Autodesk Inventor part; units mm, degrees
ref_plane "YZ Plane" through (0, 0, 0) normal (1, 0, 0) x (0, 1, 0)
ref_plane "XZ Plane" through (0, 0, 0) normal (0, 1, 0) x (-1, 0, 0)
ref_plane "XY Plane" through (0, 0, 0) normal (0, 0, 1) x (1, 0, 0)
sketch "Sketch1" plane through (0, 0, 0) normal (0, 0, 1) x (1, 0, 0)
  circle A0 centre (0, 0) radius 2.3241
  line L0 (0, 0) -> (12.7, 0)
  circle A1 centre (12.7, 0) radius 2.3241
  line L1 (0, 0) -> (12.7, 0) construction
  line L2 (0, -6.35) -> (12.7, -6.35)
  line L3 (12.7, 6.35) -> (0, 6.35)
  arc A2 (0, 6.35) -> (0, -6.35) centre (0, 0) ccw
  arc A3 (12.7, -6.35) -> (12.7, 6.35) centre (12.7, 0) ccw
  point P0 (6.35, 0)
  dimension "d0" = 4.6482
  dimension "d1" = 12.7
  dimension "d2" = 4.6482
  dimension "d3" = 12.7
extrude "Extrusion1" add sketch "Sketch1" along normal blind 12.7
sketch "Sketch2" plane through (0, 0, 0) normal (0, 0, -1) x (-1, 0, 0)
  circle A0 centre (-12.7, 0) radius 2.3241
  circle A1 centre (0, 0) radius 2.3241
  circle A2 centre (-12.7, 0) radius 4.1275
  circle A3 centre (0, 0) radius 4.1275
  dimension "d6" = 8.255
  dimension "d7" = 8.255
extrude "Extrusion2" cut sketch "Sketch2" against normal blind 2.54
sketch "Sketch3" plane through (0, 0, 12.7) normal (0, 0, 1) x (1, 0, 0)
  arc A0 (0, 6.35) -> (0, -6.35) centre (0, 0) ccw
  arc A1 (12.7, -6.35) -> (12.7, 6.35) centre (12.7, 0) ccw
  line L0 (12.7, 6.35) -> (0, 6.35)
  arc A2 (0, 6.35) -> (0, -6.35) centre (0, 0) ccw
  line L1 (0, -6.35) -> (12.7, -6.35)
  circle A3 centre (0, 0) radius 2.3241
  circle A4 centre (12.7, 0) radius 2.3241
  line L2 (19.05, 0) -> (19.05, 38.1)
  line L3 (-6.35, 0) -> (-6.35, 38.1)
  arc A5 (0, 6.35) -> (0, -6.35) centre (0, 0) ccw
  line L4 (-6.35, 38.1) -> (19.05, 38.1)
  line L5 (-6.35, 38.1) -> (-69.85, 38.1)
  line L6 (-6.35, 38.1) -> (-72.261, 62.0897)
  line L7 (-72.261, 62.0897) -> (-72.261, 49.3897)
  arc A6 (-6.35, 0) -> (-72.261, 49.3897) centre (-100.4419, -56.8924) ccw
  line L8 (-34.5064, 31.0993) -> (-34.5064, 48.3481)
  line L9 (-45.0661, 38.1) -> (-45.0661, 52.1915)
  point P0 (0, 6.35)
  point P1 (-34.5064, 38.1)
  dimension "d10" = 38.1
  dimension "d14" = 63.5
  dimension "d15" = 20
  dimension "d16" = 12.7
extrude "Extrusion3" add sketch "Sketch3" against normal up to surface (12.7 mm away) contours A0 L3 L4 L2 A1 L0 | A6 L8 L5 L3 | L5 L8 L6
fillet "Fillet1" radius 6.35 1 edges at (19.05, 38.1, 6.35)
fillet "Fillet2" radius 101.6 1 edges at (-6.35, 38.1, 6.35)
extrude "Extrusion7" add sketch "Sketch3" against normal blind 12.7 contours A0 L3 L4 L2 A1 L0 | A6 L8 L5 L3 | A6 L5 L8 | L5 L9 L6 L8
fillet "Fillet3" radius 6.35 3 edges at (-45.0661, 52.1915, 6.35) (-45.0661, 38.1, 6.35) (19.05, 38.1, 6.35)
sketch "Sketch6" plane through (0, 0, 12.7) normal (0, 0, 1) x (1, 0, 0)
  line L0 (-36.5443, 49.0898) -> (-23.1844, 44.2272)
  line L1 (-26.9453, 41.2324) -> (-18.0387, 37.9907)
  arc A0 (-23.1844, 44.2272) -> (11.5648, 38.1) centre (11.5648, 139.7) ccw
  arc A1 (-18.0387, 37.9907) -> (5.1275, 33.9059) centre (5.1275, 101.6392) ccw
  arc A2 (-36.5443, 49.0898) -> (-45.0661, 43.1228) centre (-38.7161, 43.1228) ccw
  arc A3 (-26.9453, 41.2324) -> (-32.6265, 37.2544) centre (-28.3931, 37.2544) ccw
  arc A4 (-45.0661, 41.681) -> (-42.0862, 36.2991) centre (-38.7161, 41.681) ccw
  arc A5 (-32.6265, 36.2932) -> (-30.6399, 32.7052) centre (-28.3932, 36.2932) ccw
  line L2 (-45.0661, 41.681) -> (-45.0661, 43.1228)
  line L3 (-32.6265, 36.2932) -> (-32.6265, 37.2544)
  arc A6 (-6.35, 0) -> (0, -6.35) centre (0, 0) ccw
  arc A7 (-6.8158, 8.5058) -> (-30.6399, 32.7052) centre (-69.5437, -29.4224) ccw
  arc A8 (12.7, -6.35) -> (19.05, 0) centre (12.7, 0) ccw
  line L4 (-6.8158, 8.5058) -> (10.1176, 8.5058)
  line L5 (10.1176, 8.5058) -> (10.1176, 30.026)
  line L6 (12.7, 38.1) -> (11.5648, 38.1)
  line L7 (5.1275, 33.9059) -> (5.8843, 33.9059)
  arc A9 (10.1176, 30.026) -> (5.8843, 33.9059) centre (5.8784, 29.65) ccw
  circle A10 centre (-38.7161, 43.1228) radius 3.5825
  line L8 (-30.6399, 32.7052) -> (-41.3753, 40.7221)
  line L9 (-37.1542, 46.3469) -> (-25.5432, 40.7221)
  line L10 (-6.8158, 8.5058) -> (-5.0194, 5.3621)
  line L11 (-5.0194, 5.3621) -> (15.0904, 5.3621)
  line L12 (15.0904, 5.3621) -> (15.0904, 31.7435)
  line L13 (15.0904, 31.7435) -> (5.8842, 33.9059)
  point P0 (5.8842, 33.9059)
extrude "Extrusion8" cut sketch "Sketch6" against normal blind 12.7 contours A3 L3 A5 L8 A10 L9 L1 | L1 A1 L7 L13 A9 L5 L4 A7 L8 A5 L3 A3 | A10 L8 | L13 L12 L11 L10 L4 L5 A9 picked at (-38.0775, 41.7353)
fillet "Fillet4" radius 6.35 4 edges at (15.0904, 31.7435, 6.35) (5.8842, 33.9059, 6.35) (-5.0194, 5.3621, 6.35) (15.0904, 5.3621, 6.35)
sketch "Sketch7" plane through (0, 0, 12.7) normal (0, 0, 1) x (1, 0, 0)
  point P0 (0, 0)
sketch "Sketch8" plane through (0, 0, 12.7) normal (0, 0, 1) x (1, 0, 0)
  arc A0 (-6.8158, 8.5058) -> (-30.6399, 32.7052) centre (-69.5437, -29.4224) ccw
  line L0 (-30.6399, 32.7052) -> (5.4461, 34.0088)
  line L1 (5.4461, 34.0088) -> (12.4378, 32.3666)
  line L2 (10.1924, 32.894) -> (6.6005, 33.7376)
  line L3 (12.4378, 32.3666) -> (-28.2224, 30.8977)
  line L4 (-28.2224, 30.8977) -> (-30.6399, 32.7052)
  arc A1 (8.7404, 5.3621) -> (15.0904, 11.7121) centre (8.7404, 11.7121) ccw
  line L5 (8.7404, 5.3621) -> (-31.9338, 43.818)
  line L6 (-25.5432, 40.7221) -> (-37.1542, 46.3469)
  line L7 (11.702, 6.0501) -> (-26.744, 42.3992)
  line L8 (-26.744, 42.3992) -> (-31.9338, 43.818)
  point P0 (0, 0)
  point P1 (-20.565, 33.0692)
  point P2 (-18.6346, 31.2441)
  point P3 (11.6714, 6.079)
  point P4 (-15.0811, 31.3725)
  point P5 (-17.0115, 33.1975)
extrude "Extrusion9" add sketch "Sketch8" against normal blind 12.7
fillet "Fillet5" radius 1.5875 8 edges at (-15.0811, 31.3725, 6.35) (-27.9088, 30.9091, 6.35) (-20.565, 33.0692, 6.35) (-30.6399, 32.7052, 6.35) (8.7404, 5.3621, 6.35) (11.6714, 6.079, 6.35) (-18.6346, 31.2441, 6.35) (-17.0115, 33.1975, 6.35)
fillet "Fillet6" radius 0.7937 1 edges at (-24.6115, 40.383, 6.35)
fillet "Fillet7" radius 0.3969 1 edges at (3.2884, 33.9309, 6.35)
properties part number "Ring Bay"
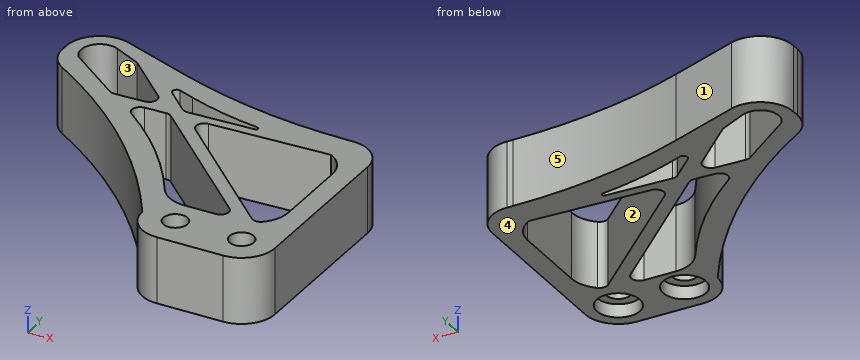
The model under review builds one solid part; all positions refer to its coordinate system, in mm. Face numbers are marked on the shaded views. A direction names the side the tool comes from. Give positions to 0.01 mm unless a question says otherwise; leave off trailing zeros. Loops run counter-clockwise (first coordinate to the right, second up) from the corner with the lowest first, then second, coordinate; pieces in that order, holes last. Notation, with made-up numbers: (84, -16.5) -> (101, -16.5) arc R25 cw to (101, 9.5) -> close; hole circle Ø3 at (-17, 21.25). An arc over 180 degrees is marked (long way). Put each result on its own line as item: value. Start each with the question number.
1. We need section D-D on z = 7. State how many separate pieces and enclosed holes the cut face has, then the cut area to 3 significant figures.
2. For the marked faces 1 and 2, list the 3-axis set-ups (+Z, -Z, +X, -X, +Y, -Y) from which the entire face can be reached by the end or side of a thin tool; tool diameter is ignored.
3. We need section C-C on x = -27. State the section outline as (y, z) points.
4. We need section A-A on x = -15. State the section outline as (y, z) points.
5. Mouldability with a two-part tool opening along X and no side actions: class the marked faces 3, 4 and 5 as released by +X, released by -X, zero draft, split by the parting line, or undercut.
6. Clearance check with flat-ended pins moving along their axes: P1, Ø6, axis at y = 35.5, z = 7, coming from the +X side; P2, Ø5, axis at y = 2, z = 8, coming from the -X side; P3, Ø1.5, axis at x = -16.5, z = 4.5, coming from the +Y side. State where each tip first meets the part, or that it passes through.
7. Wall thickness on probe 1 along X at (y, z) = (0, 8.25); probe 2 along Y at (x, z) = (12.7, 1.05); probe 3 along Y at (x, z) = (12.7, 8.25): over which ranges is each line inside the solid? List them lowest first.
8. We need section B-B on y = 18. State the section outline as (x, z) points, then the cut area to 3 significant figures.
Determined:
1. separate pieces: 1
1. enclosed holes: 6
1. area: 1,090 mm^2
2. face 1: +Z, -Z, +X, +Y
2. face 2: +Z, -Z
3. outline: (24.94, 0) -> (32.84, 0) -> (32.84, 12.7) -> (24.94, 12.7) -> close; (39.15, 0) -> (45.62, 0) -> (45.62, 12.7) -> (39.15, 12.7) -> close
4. outline: (12.32, 0) -> (19.55, 0) -> (19.55, 12.7) -> (12.32, 12.7) -> close; (27.81, 0) -> (33.27, 0) -> (33.27, 12.7) -> (27.81, 12.7) -> close; (36.97, 0) -> (41.63, 0) -> (41.63, 12.7) -> (36.97, 12.7) -> close
5. face 3: undercut
5. face 4: zero draft
5. face 5: released by +X
6. P1: x = 19.01
6. P2: x = -9.22
6. P3: y = 42.27
7. probe 1: -6.35 to -2.32, 2.32 to 10.38, 15.02 to 19.05
7. probe 2: -6.35 to -4.13, 4.13 to 6.76, 31.68 to 38.1
7. probe 3: -6.35 to -2.32, 2.32 to 6.76, 31.68 to 38.1
8. outline: (-19.94, 0) -> (-13.65, 0) -> (-13.65, 12.7) -> (-19.94, 12.7) -> close; (-4.63, 0) -> (-0.94, 0) -> (-0.94, 12.7) -> (-4.63, 12.7) -> close; (15.09, 0) -> (19.05, 0) -> (19.05, 12.7) -> (15.09, 12.7) -> close
8. area: 177 mm^2
